Part model, mm, in its own coordinate system. A direction names the side the tool comes from. Give positions to 0.01 mm unless a question says otherwise; leave off trailing zeros. Write each loop counter-clockwise with the first axis right and the second up, starting at its lowest first coordinate (ties: lowest second). Pieces come first, ordered by that corner, then holes. Notation, with made-up numbers: M -1.75,9 L 12.25,9 A17 cw 12.25,42 Z; hole C -35,-11 d9. An arc over 180 degrees is marked long. Use a Markdown table: item, result.
```python
from build123d import *

# Parameters (mm, degrees)
SKETCH_W     = 27
SKETCH_H     = 9
PAD_DEPTH    = 6.5
CHAMFER_SIZE = 1


with BuildPart() as part:
    # Sketch → Pad (new body)
    with BuildSketch(Plane.XY):
        Rectangle(SKETCH_W, SKETCH_H)
        with BuildLine():
            ThreePointArc((-6, 1.7), (-7.7, 0), (-6, -1.7))
            Line((-6, -1.7), (6, -1.7))
            ThreePointArc((6, -1.7), (7.7, 0), (6, 1.7))
            Line((-6, 1.7), (6, 1.7))
        make_face(mode=Mode.SUBTRACT)
    extrude(amount=PAD_DEPTH)

    # Chamfer
    chamfer_edges = [part.edges().sort_by_distance(p)[0] for p in [
        (0, -4.5, 6.5),
        (0, 4.5, 6.5),
    ]]
    chamfer(chamfer_edges, length=CHAMFER_SIZE)


solid = part.part
```
1. Cut at A-A, the plane y = 0. Give the cut face in (x, z), then the cut area to 3 significant figures.
Findings below:
| item | result |
|---|---|
| outline | M -13.5,0 L -7.7,0 L -7.7,6.5 L -13.5,6.5 Z; M 7.7,0 L 13.5,0 L 13.5,6.5 L 7.7,6.5 Z |
| area | 75.4 mm2 |
2. Cut at C-C, the plane z = 2. Give the cut face in (x, y).
Findings below:
| item | result |
|---|---|
| outline | M -13.5,-4.5 L 13.5,-4.5 L 13.5,4.5 L -13.5,4.5 Z; hole M -6,-1.7 L 6,-1.7 A1.7 ccw 6,1.7 L -6,1.7 A1.7 ccw Z |
3. Cut at B-B, the plane z = 6.25. Give the cut face in (x, y).
Findings below:
| item | result |
|---|---|
| outline | M -13.5,-3.75 L 13.5,-3.75 L 13.5,3.75 L -13.5,3.75 Z; hole M -6,-1.7 L 6,-1.7 A1.7 ccw 6,1.7 L -6,1.7 A1.7 ccw Z |
4. Drill centre lines: L1, parallel to Y at x = -5, z = 4.75; L2, parallel to X at y = -0.75, z = 4; L3, parallel to Y at x = 7, z = 1.5. Where is each one in solid material? Low to high.
Findings below:
| item | result |
|---|---|
| L1 | -4.5 to -1.7, 1.7 to 4.5 |
| L2 | -13.5 to -7.53, 7.53 to 13.5 |
| L3 | -4.5 to -1.37, 1.37 to 4.5 |
5. Two-plate mould, pull along X, no slides. Class faces 3 (the flat face through (0, -1.7, 3)), 4 (the flat face through (0, 2, 0)), 5 (the flat face through (13.5, 0, 3)): released by +X, released by -X, zero draft, split by the parting line, or undercut.
Findings below:
| item | result |
|---|---|
| face 3 | undercut |
| face 4 | zero draft |
| face 5 | released by +X |
6. Cut at D-D, the plane y = 4. Give the cut face in (x, z), then the cut area to 3 significant figures.
Findings below:
| item | result |
|---|---|
| outline | M -13.5,0 L 13.5,0 L 13.5,6 L -13.5,6 Z |
| area | 162 mm2 |
7. Tool access for faces 1 (the cylindrical face through (-7.7, 0, 3.2)), 2 (the flat face through (0, -4.5, 3)): list every direction of +Z, -Z, +X, -X, +Y, -Y with a clear straight run to the whole face (end or side of a thin tool).
Findings below:
| item | result |
|---|---|
| face 1 | +Z, -Z |
| face 2 | +Z, -Z, +X, -X, -Y |
